Design review of the part built by this model. Coordinates are the model's own, in mm. A direction names the side the tool comes from. Coordinates: 2 decimals unless noted, no trailing zeros. Loops run counter-clockwise (first coordinate to the right, second up) from the corner with the lowest first, then second, coordinate; pieces in that order, holes last. Notation, with made-up numbers: M 5,21 L 61,21 A31 cw 61,49 Z; hole C 59.5,-10 d6. An arc over 180 degrees is marked long. Put each result on its own line as item: value. Start each with the question number.
(1) For probe 1 along Y at (x, z) = (74.5, 4.7); probe 2 along Z at (x, y) = (-86.1, -31.25); probe 3 along Z at (x, y) = (-59, 9), list the stretches that pass through material, from the lowest coordinate up. Write a range as [from, to].
(2) Take a section at B-B, the plane y = 20. Give the boundary of the cut face in (x, z), then the cut area to 3 significant figures.
(3) For faces 1 (the flat face through (2, 1, 6)), 2 (the cylindrical face through (21.76, 30.33, 2.96)), list the 3-axis set-ups (+Z, -Z, +X, -X, +Y, -Y) from which the entire face can be reached by the end or side of a thin tool; tool diameter is ignored.
(4) Take a section at C-C, the plane z = 8. Give the boundary of the cut face in (x, y), then the cut area to 3 significant figures.
(5) Take a section at D-D, the plane x = -24. Give the boundary of the cut face in (y, z), then the cut area to 3 significant figures.
(6) Clearance check with flat-ended pins moving along their axes: pin 1 (12 mm diameter, centred on y = 0, z = 18, fed in from +X); pin 2 (5 mm diameter, centred on x = 29, y = 10, fed in from +Z); pin 3 (1 mm diameter, centred on y = -17, z = 20.5, fed in from -X); pin 4 (2.5 mm diameter, centred on x = 22.5, y = 31.75, fed in from -Z). State where each tip first meets the part, or that it passes through.
(7) Take a section at A-A, the plane x = 22.5. Give the boundary of the cut face in (y, z).
(8) The part is to be moulded in two halves that separate along X. For faces 3 (the cylindrical face through (47.02, 31.14, 2.96)), 4 (the flat face through (-85, 1, 25)), 5 (the cylindrical face through (72.974, -31.269, 2.958)), 6 (the flat face through (-87.5, -1, 23)), say which applies: +X half, -X half, draft (parallel to the pull), parting line (faces both ways), or undercut.
```python
from build123d import *

# Parameters (mm, degrees)
F0_W     = 175
F0_H     = 72.5
F1_DEPTH = 25
F2_W     = 169
F2_H     = 72.5
F3_DEPTH = 19
F5_D     = 3.2
F6_W     = 72.5
F6_H     = 2
F7_DEPTH = 2
F9_D     = 2


with BuildPart() as f1:
    # F0 (on Top) → F1 (new body)
    with BuildSketch(Plane.XY):
        Rectangle(F0_W, F0_H)
    extrude(amount=F1_DEPTH)

    # F2 (on face) → F3 (cut)
    with BuildSketch(Plane.XY.offset(25)):
        with Locations((3, 0)):
            Rectangle(F2_W, F2_H)
    extrude(amount=-F3_DEPTH, mode=Mode.SUBTRACT)

    # F5 (through all)
    with Locations(Plane.XY.offset(6)):
        with Locations((22.5, 31.75), (48.5, 31.75), (74.5, 31.75), (74.5, -31.75), (48.5, -31.75), (22.5, -31.75)):
            Hole(F5_D / 2)

    # F6 (on face) → F7 (cut)
    with BuildSketch(Plane(origin=(-87.5, 0, 0), x_dir=(0, -1, 0), z_dir=(-1, 0, 0))):
        with Locations((0, 5)):
            Rectangle(F6_W, F6_H)
        with Locations((0, 20.8)):
            Rectangle(F6_W, F6_H)
    extrude(amount=-F7_DEPTH, mode=Mode.SUBTRACT)

    # F9 (through all)
    with Locations(Plane(origin=(-87.5, 0, 0), x_dir=(0, -1, 0), z_dir=(-1, 0, 0))):
        with Locations((-31.25, 12.9), (-11.25, 12.9), (11.25, 12.9), (31.25, 12.9)):
            Hole(F9_D / 2)


solid = f1.part
```
Computed values:
1. probe 1: y = [-36.25, -33.35], [-30.15, 30.15], [33.35, 36.25]
1. probe 2: z = [0, 4], [6, 11.9], [13.9, 19.8], [21.8, 25]
1. probe 3: z = [0, 6]
2. outline: M -87.5,0 L 87.5,0 L 87.5,6 L -81.5,6 L -81.5,25 L -87.5,25 L -87.5,21.8 L -85.5,21.8 L -85.5,19.8 L -87.5,19.8 L -87.5,6 L -85.5,6 L -85.5,4 L -87.5,4 Z
2. area: 1,160 mm^2
3. face 1: +Z, +X, +Y, -Y
3. face 2: +Z, -Z
4. outline: M -87.5,-36.25 L -81.5,-36.25 L -81.5,36.25 L -87.5,36.25 Z
4. area: 435 mm^2
5. outline: M -36.25,0 L 36.25,0 L 36.25,6 L -36.25,6 Z
5. area: 435 mm^2
6. pin 1: stops at x = -81.5
6. pin 2: stops at z = 6
6. pin 3: stops at x = -85.5
6. pin 4: passes through
7. outline: M -36.25,0 L -33.35,0 L -33.35,6 L -36.25,6 Z; M -30.15,0 L 30.15,0 L 30.15,6 L -30.15,6 Z; M 33.35,0 L 36.25,0 L 36.25,6 L 33.35,6 Z
8. face 3: undercut
8. face 4: draft
8. face 5: undercut
8. face 6: -X half
